Read the model definition and answer for the solid it produces. Units are mm, in the model's axes. A direction names the side the tool comes from. Round coordinates to 2 decimals unless told otherwise and drop trailing zeros. Write each loop counter-clockwise with the first axis right and the second up, starting at its lowest first coordinate (ties: lowest second). Pieces come first, ordered by that corner, then holes. Notation, with made-up numbers: (-40, 48) -> (19, 48) arc R23 ccw to (19, 76) -> close; hole circle Ø3 at (-30.5, 50.25). An arc over 180 degrees is marked (long way). Return JSON: item names as keys, results as strings.
from build123d import *

# Parameters (mm, degrees)
BOSS_EXTRUDE1_DEPTH          = 22.225
F_10_0_1935_DIAMETER_HOLE1_D = 4.9149


with BuildPart() as part:
    # Sketch1 → Boss-Extrude1 (new, symmetric)
    with BuildSketch(Plane(origin=(0, 0, 0), x_dir=(0, 0, -1), z_dir=(1, 0, 0))):
        Polygon((0, 0), (44.45, 0), (44.45, 44.45), (38.1, 44.45), (38.1, 6.35), (0, 6.35), align=None)
    extrude(amount=BOSS_EXTRUDE1_DEPTH, both=True)

    # #10 (0.1935) Diameter Hole1 (through all)
    with Locations(Plane(origin=(0, 6.35, 0), x_dir=(1, 0, 0), z_dir=(0, 1, 0))):
        with Locations((13.470384182, 5.579615818), (-13.470384182, 32.520384182), (-13.470384182, 5.579615818), (13.470384182, 32.520384182)):
            f_10_0_1935_diameter_hole1 = Hole(F_10_0_1935_DIAMETER_HOLE1_D / 2)

    # Mirror1: #10 (0.1935) Diameter Hole1 across plane
    add(f_10_0_1935_diameter_hole1.mirror(Plane(origin=(0, 22.225, -22.225), x_dir=(0, 0.7071067811865476, 0.7071067811865475), z_dir=(0, 0.7071067811865475, -0.7071067811865476))), mode=Mode.SUBTRACT)


solid = part.part
Item 1: For a pull along Y with two mould halves and no side action, classify faces 3 (the flat face through (0, 22, -44.45)), 4 (the flat face through (0, 6.35, -19)), 5 (the cylindrical face through (-12.94, 41.27, -41.32)), 6 (the cylindrical face through (-13.15, 9.493, -41.319)) as released by +Y, released by -Y, zero draft, split by the parting line, or undercut.
Worked answers:
{"face 3": "zero draft", "face 4": "released by +Y", "face 5": "undercut", "face 6": "undercut"}
Item 2: Section C-C (y = 40.5) is taken. Give the vertices of the cut face in (x, z) (3 decimals).
Worked answers:
{"outline": "(-22.225, -44.45) -> (-15.31, -44.45) -> (-15.31, -38.1) -> (-22.225, -38.1) -> close; (-11.631, -44.45) -> (11.631, -44.45) -> (11.631, -38.1) -> (-11.631, -38.1) -> close; (15.31, -44.45) -> (22.225, -44.45) -> (22.225, -38.1) -> (15.31, -38.1) -> close"}
Item 3: A tool of negligible diameter and unlimited length cuts with its end or side. For faces 1 (the flat face through (0, 26, -38.1)), 2 (the cylindrical face through (14, 41.27, -41.32)), from which of +Z, -Z, +X, -X, +Y, -Y can it reach the whole face along a straight path? Write none if from no direction.
Worked answers:
{"face 1": "+Z, +X, -X, +Y", "face 2": "+Z, -Z"}
Item 4: Straight lines are drawn through the part: L1, parallel to Y at x = -12, z = -39.5; L2, parallel to Z at x = -15, y = 18; L3, parallel to Y at x = 12, z = -27.5. For each, find the intervals that lie inside material, in ascending order. Write a range as [from, to].
Worked answers:
{"L1": "y = [0, 9.96], [13.9, 36.9], [40.84, 44.45]", "L2": "z = [-44.45, -38.1]", "L3": "y = [0, 6.35]"}
Item 5: Section B-B (y = 3) is taken. Give the vertices of the cut face in (x, z) (3 decimals).
Worked answers:
{"outline": "(-22.225, -44.45) -> (22.225, -44.45) -> (22.225, 0) -> (-22.225, 0) -> close; hole circle Ø4.915 at (-13.47, -32.52); hole circle Ø4.915 at (-13.47, -5.58); hole circle Ø4.915 at (13.47, -32.52); hole circle Ø4.915 at (13.47, -5.58)"}
Item 6: Section A-A (x = 15) is taken. Give the vertices of the cut face in (y, z), then the cut area to 3 significant figures.
Worked answers:
{"outline": "(0, -44.45) -> (10.01, -44.45) -> (10.01, -38.1) -> (6.35, -38.1) -> (6.35, -34.44) -> (0, -34.44) -> close; (0, -30.6) -> (6.35, -30.6) -> (6.35, -7.5) -> (0, -7.5) -> close; (0, -3.66) -> (6.35, -3.66) -> (6.35, 0) -> (0, 0) -> close; (13.85, -44.45) -> (36.95, -44.45) -> (36.95, -38.1) -> (13.85, -38.1) -> close; (40.79, -44.45) -> (44.45, -44.45) -> (44.45, -38.1) -> (40.79, -38.1) -> close", "area": "426 mm2"}
Item 7: Section D-D (z = -40) is taken. Give the vertices of the cut face in (x, y) (3 decimals).
Worked answers:
{"outline": "(-22.225, 0) -> (22.225, 0) -> (22.225, 44.45) -> (-22.225, 44.45) -> close; hole circle Ø4.915 at (-13.47, 11.93); hole circle Ø4.915 at (-13.47, 38.87); hole circle Ø4.915 at (13.47, 11.93); hole circle Ø4.915 at (13.47, 38.87)"}
Item 8: Flat-ended cylindrical pins translate along their axes: pin 1 (5.5 mm diameter, centred on x = 13.47, z = -5.58, fed in from +Y); pin 2 (3 mm diameter, centred on x = 7, z = -6, fed in from -Y); pin 3 (1.5 mm diameter, centred on x = 5.5, y = 33.5, fed in from +Z). Find the tip coordinate at first contact, or state that the pin passes through.
Worked answers:
{"pin 1": "stops at y = 6.35", "pin 2": "stops at y = 0", "pin 3": "stops at z = -38.1"}
